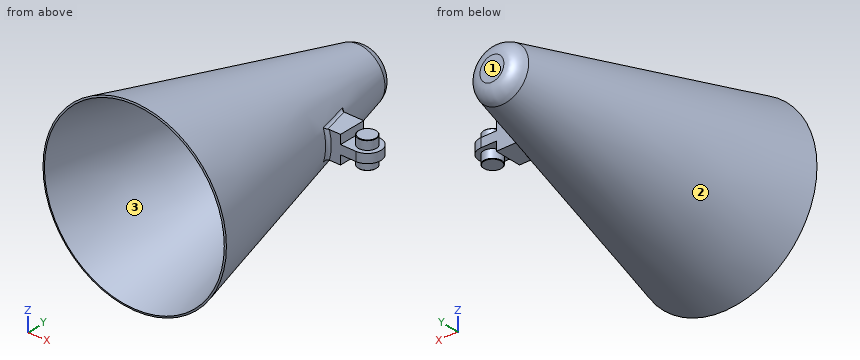
from build123d import *

# Parameters (mm, degrees)
BOSS_EXTRUDE1_REACH = 406.646
BOSS_EXTRUDE1_START = 70
SKETCH3_W           = 30
SKETCH3_H           = 30
BOSS_EXTRUDE2_DEPTH = 5
SKETCH5_R           = 10
BOSS_EXTRUDE3_DEPTH = 15
FILLET1_R           = 3
CHAMFER1_SIZE       = 0.5


with BuildPart() as part:
    # Sketch2 → Revolve-Thin1 (revolve)
    with BuildSketch(Plane.XY, mode=Mode.PRIVATE) as revolve_thin1_sk:
        with BuildLine():
            Line((0, 300), (-13.288353904, 300))
            ThreePointArc((-13.288353904, 300), (-22.519537045, 296.82308157), (-27.840491406, 288.638034376))
            Line((-27.840491406, 288.638034376), (-100, 0))
            Line((-100, 0), (-101.940285, 0.48507125))
            Line((-101.940285, 0.48507125), (-29.780776406, 289.123105626))
            ThreePointArc((-29.780776406, 289.123105626), (-23.750361464, 298.399492446), (-13.288353904, 302))
            Line((-13.288353904, 302), (0, 302))
            Line((0, 302), (0, 300))
        make_face()
    revolve(revolve_thin1_sk.sketch.rotate(Axis((0, 0, 0), (0, 1, 0)), 270), axis=Axis((0, 0, 0), (0, 1, 0)))

    # Sketch3 → Boss-Extrude1 (add, up to next)
    with BuildSketch(Plane(origin=(0, 0, 0), x_dir=(0, 0, -1), z_dir=(1, 0, 0)).offset(BOSS_EXTRUDE1_START), mode=Mode.PRIVATE) as boss_extrude1_sk1:
        with Locations((0, 200)):
            Rectangle(SKETCH3_W, SKETCH3_H)
    boss_extrude1_tool1 = extrude(boss_extrude1_sk1.sketch, amount=-BOSS_EXTRUDE1_REACH, mode=Mode.PRIVATE) - part.part
    add(boss_extrude1_tool1.solids().sort_by_distance((70, 200, 0))[0])

    # Sketch4 → Boss-Extrude2 (add, symmetric)
    with BuildSketch(Plane.XY):
        with BuildLine():
            Line((70, 215), (87, 215))
            ThreePointArc((87, 215), (102, 200), (87, 185))
            Line((87, 185), (70, 185))
            Line((70, 185), (70, 215))
        make_face()
    extrude(amount=BOSS_EXTRUDE2_DEPTH, both=True)

    # Sketch5 → Boss-Extrude3 (add, symmetric)
    with BuildSketch(Plane.XY):
        with Locations(Location((87, 200, 0), (0, 0, 180))):
            Circle(SKETCH5_R)
    extrude(amount=BOSS_EXTRUDE3_DEPTH, both=True)

    # Fillet1
    fillet1_edges = [part.edges().sort_by_distance(p)[0] for p in [
        (48.311552813, 215, 0),
        (49.853019013, 200.003141557, -15),
        (49.853019013, 200.003141557, 15),
        (55.811552813, 185, 0),
    ]]
    fillet(fillet1_edges, radius=FILLET1_R)

    # Chamfer1
    chamfer1_edges = [part.edges().sort_by_distance(p)[0] for p in [
        (97, 200, -15),
        (97, 200, 15),
    ]]
    chamfer(chamfer1_edges, length=CHAMFER1_SIZE)


solid = part.part
Geometry: final body of the model. Coordinates: model frame, mm. Face numbers are marked on the shaded views. Round coordinates to 2 decimals unless told otherwise and drop trailing zeros. Loops run counter-clockwise (first coordinate to the right, second up) from the corner with the lowest first, then second, coordinate; pieces in that order, holes last. Notation, with made-up numbers: M -3,39 L 6,39 A26 cw 6,72 Z; hole C -36.75,58 d3. An arc over 180 degrees is marked long. Put each result on its own line as item: value. Start each with the question number.
(1) Contact query for flat-ended pins moving along their axis: pin 1 Ø9 at (x, y) = (82, 196.5) entering from -Z; pin 2 Ø6 at (x, z) = (-9, 2.5) entering from -Y; pin 3 Ø6.5 at (x, y) = (62.5, 206.5) entering from +Z. Output: stop coordinate, or through.
(2) Material intervals for line 1 along X through (y, z) = (193, 12); line 2 along X through (y, z) = (155.5, -11.5); line 3 along Z through (x, y) = (-67, 23), sorted ascending. Write a range as [from, to].
(3) Section query B-B (y = 272). Return loops of the section in (x, z).
(4) Draft query along X for the marked faces 1, 2 and 3. Return one class per face: +X half, -X half, draft (parallel to the pull), parting line (faces both ways), or undercut.
(5) Section query A-A (y = 173). Return loops of the section in (x, z).
Findings below:
1. pin 1: stops at z = -15
1. pin 2: stops at y = 300
1. pin 3: stops at z = 15
2. line 1: x = [-52.46, -50.34], [50.34, 70], [79.86, 94.14]
2. line 2: x = [-62.13, -60.03], [60.03, 62.13]
2. line 3: z = [-69.19, -66.29], [66.29, 69.19]
3. outline: C 0,0 d68.12; hole C 0,0 d64
4. face 1: draft
4. face 2: parting line
4. face 3: undercut
5. outline: C 0,0 d117.62; hole C 0,0 d113.5
